Can you work these out from the model? Positions are in its coordinate system, mm. Coordinates: 2 decimals unless noted, no trailing zeros. Order: outer loops, then holes, each group sorted by start corner. A loop starts at its lowest first (then second) coordinate and runs counter-clockwise, first axis right, second up. Notation, with made-up numbers: (40.25, 46) -> (96.25, 46) arc R26 cw to (96.25, 65) -> close; hole circle Ø2 at (8.5, 11). An arc over 180 degrees is marked (long way). Return JSON: item names as keys, results as strings. Group by question number.
1) If we section it at B-B, the plane z = 9.25: Please give me the cut outline in (x, y), then the cut area to 3 significant figures.
2) If we section it at C-C, the plane y = 86: Please give me the cut outline in (x, z), then the cut area to 3 significant figures.
3) If I drill on probe 1 along X at (y, z) = (63, 11.5); probe 2 along X at (y, z) = (66.5, 8.25); probe 3 along Y at (x, z) = (18.5, 4.5), over which ranges is the centre line in solid material (lowest first)? Write a range as from..to.
4) If we section it at A-A, the plane y = 70: Please give me the cut outline in (x, z).
5) If we section it at D-D, the plane x = 30: Please give me the cut outline in (y, z).
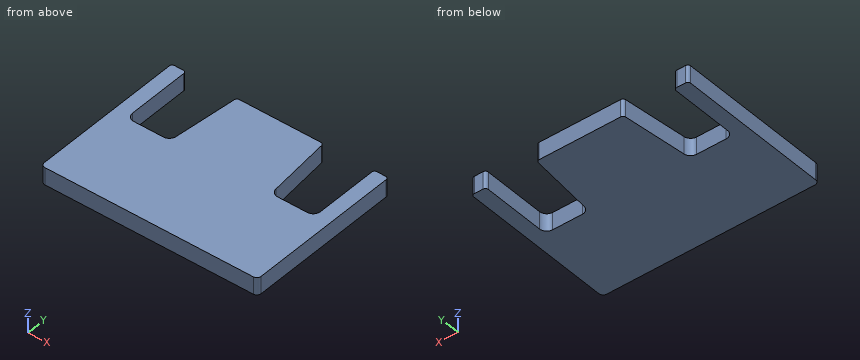
from build123d import *

# Parameters (mm, degrees)
ESQUISSE1_W                  = 150
ESQUISSE1_H                  = 110
BOSS_EXTRU_1_DEPTH           = 12
ENL_V_MAT_EXTRU_1_DEPTH      = 187.397424875
ENL_V_MAT_EXTRU_1_DEPTH_BACK = 187.397424875
CONG_1_R                     = 5
CONG_2_R                     = 2
CONG_3_R                     = 3


with BuildPart() as part:
    # Esquisse1 → Boss.-Extru.1 (new body)
    with BuildSketch(Plane.XY):
        with Locations((75, 55)):
            Rectangle(ESQUISSE1_W, ESQUISSE1_H)
    extrude(amount=BOSS_EXTRU_1_DEPTH)

    # Esquisse2 → Enlèv. mat.-Extru.1 (cut, two sides: drawn at the far end of the back side and taken through both)
    with BuildSketch(Plane.XY.offset(12).offset(-ENL_V_MAT_EXTRU_1_DEPTH_BACK)):
        Polygon((105, 110), (110, 60), (140, 60), (140, 110), align=None)
        Polygon((10, 110), (45, 110), (40, 60), (10, 60), align=None)
    extrude(amount=ENL_V_MAT_EXTRU_1_DEPTH + ENL_V_MAT_EXTRU_1_DEPTH_BACK, mode=Mode.SUBTRACT)

    # Congé1
    cong_1_edges = [part.edges().sort_by_distance(p)[0] for p in [
        (10, 60, 6),
        (40, 60, 6),
        (140, 60, 6),
        (110, 60, 6),
    ]]
    fillet(cong_1_edges, radius=CONG_1_R)

    # Congé2
    cong_2_edges = [part.edges().sort_by_distance(p)[0] for p in [
        (10, 110, 6),
        (45, 110, 6),
        (105, 110, 6),
        (140, 110, 6),
        (0, 110, 6),
        (150, 110, 6),
    ]]
    fillet(cong_2_edges, radius=CONG_2_R)

    # Congé3
    cong_3_edges = [part.edges().sort_by_distance(p)[0] for p in [
        (150, 0, 6),
        (0, 0, 6),
    ]]
    fillet(cong_3_edges, radius=CONG_3_R)


solid = part.part
Result sheet:
{
 "1": {"outline": "(0, 3) arc R3 ccw to (3, 0) -> (147, 0) arc R3 ccw to (150, 3) -> (150, 108) arc R2 ccw to (148, 110) -> (142, 110) arc R2 ccw to (140, 108) -> (140, 65) arc R5 cw to (135, 60) -> (114.52, 60) arc R5 cw to (109.55, 64.5) -> (105.18, 108.2) arc R2 ccw to (103.19, 110) -> (46.81, 110) arc R2 ccw to (44.82, 108.2) -> (40.45, 64.5) arc R5 cw to (35.48, 60) -> (15, 60) arc R5 cw to (10, 65) -> (10, 108) arc R2 ccw to (8, 110) -> (2, 110) arc R2 ccw to (0, 108) -> close", "area": "13,300 mm2"},
 "2": {"outline": "(0, 0) -> (10, 0) -> (10, 12) -> (0, 12) -> close; (42.6, 0) -> (107.4, 0) -> (107.4, 12) -> (42.6, 12) -> close; (140, 0) -> (150, 0) -> (150, 12) -> (140, 12) -> close", "area": "1,020 mm2"},
 "3": {"probe 1": "x = 0..10.42, 40.06..109.94, 139.58..150", "probe 2": "x = 0..10, 40.65..109.35, 140..150", "probe 3": "y = 0..60"},
 "4": {"outline": "(0, 0) -> (10, 0) -> (10, 12) -> (0, 12) -> close; (41, 0) -> (109, 0) -> (109, 12) -> (41, 12) -> close; (140, 0) -> (150, 0) -> (150, 12) -> (140, 12) -> close"},
 "5": {"outline": "(0, 0) -> (60, 0) -> (60, 12) -> (0, 12) -> close"}
}
